Source: three-view drawing plus pictorial views. Frame: mm from the lowest corner of the part. A direction names the side the tool comes from. Coordinates: 2 decimals unless noted, no trailing zeros. Write each loop counter-clockwise with the first axis right and the second up, starting at its lowest first coordinate (ties: lowest second). Pieces come first, ordered by that corner, then holes. Notation, with made-up numbers: (-8.75, 28) -> (27.25, 28) arc R21 cw to (27.25, 32) -> close; hole circle Ø3 at (68.25, 8.5). An arc over 180 degrees is marked (long way). One line per question, with ' | ' between items. Start each with the question number.
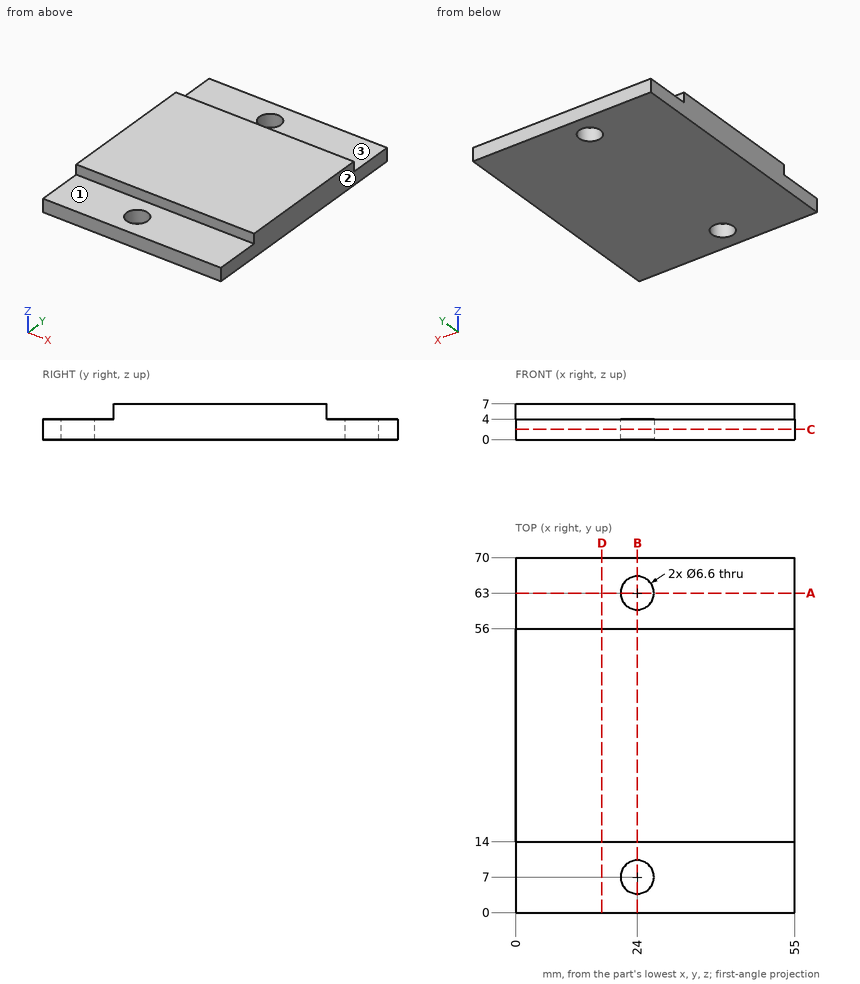
1) Section B-B, the plane x = 24. Return loops of the section in (y, z).
2) Section D-D, the plane x = 17. Return loops of the section in (y, z), then the cut area to 3 significant figures.
3) Ray query, line 1 (Y direction, x = 24, z = 3.15); line 2 (Z direction, x = 19, y = 11.5); line 3 (Y direction, x = 47.5, z = 4.5). Return the intervals inside material, ascending.
4) Section C-C, the plane z = 2. Return loops of the section in (x, y), then the cut area to 3 significant figures.
5) First-contact query: P1, Ø12, axis at x = 36, y = 18.5, coming from the -Z side; P2, Ø4, axis at x = 24, y = 63, coming from the +Z side; P3, Ø1.5, axis at x = 14.5, z = 5, coming from the -Y side; P4, Ø10.5, axis at x = 24, y = 7, coming from the +Z side. Flat tips, straight axial feed; report the tip coordinate or a pass-through.
6) Access query for the marked faces 1, 2 and 3. Directions: +Z, -Z, +X, -X, +Y, -Y. A direction counts if a zero-diameter tool reaches every point of the face in a straight line with its end or side. Return the directions, or none.
7) Section A-A, the plane y = 63. Return loops of the section in (x, z), then the cut area to 3 significant figures.
Answer block:
1) outline: (0, 0) -> (3.7, 0) -> (3.7, 4) -> (0, 4) -> close; (10.3, 0) -> (59.7, 0) -> (59.7, 4) -> (56, 4) -> (56, 7) -> (14, 7) -> (14, 4) -> (10.3, 4) -> close; (66.3, 0) -> (70, 0) -> (70, 4) -> (66.3, 4) -> close
2) outline: (0, 0) -> (70, 0) -> (70, 4) -> (56, 4) -> (56, 7) -> (14, 7) -> (14, 4) -> (0, 4) -> close | area: 406 mm2
3) line 1: y = 0 to 3.7, 10.3 to 59.7, 66.3 to 70 | line 2: z = 0 to 4 | line 3: y = 14 to 56
4) outline: (0, 0) -> (55, 0) -> (55, 70) -> (0, 70) -> close; hole circle Ø6.6 at (24, 7); hole circle Ø6.6 at (24, 63) | area: 3,780 mm2
5) P1: stops at z = 0 | P2: passes through | P3: stops at y = 14 | P4: stops at z = 4
6) face 1: +Z, +X, -X, -Y | face 2: +Z, -Z, +X, +Y, -Y | face 3: +Z, +X, -X, +Y
7) outline: (0, 0) -> (20.7, 0) -> (20.7, 4) -> (0, 4) -> close; (27.3, 0) -> (55, 0) -> (55, 4) -> (27.3, 4) -> close | area: 194 mm2
